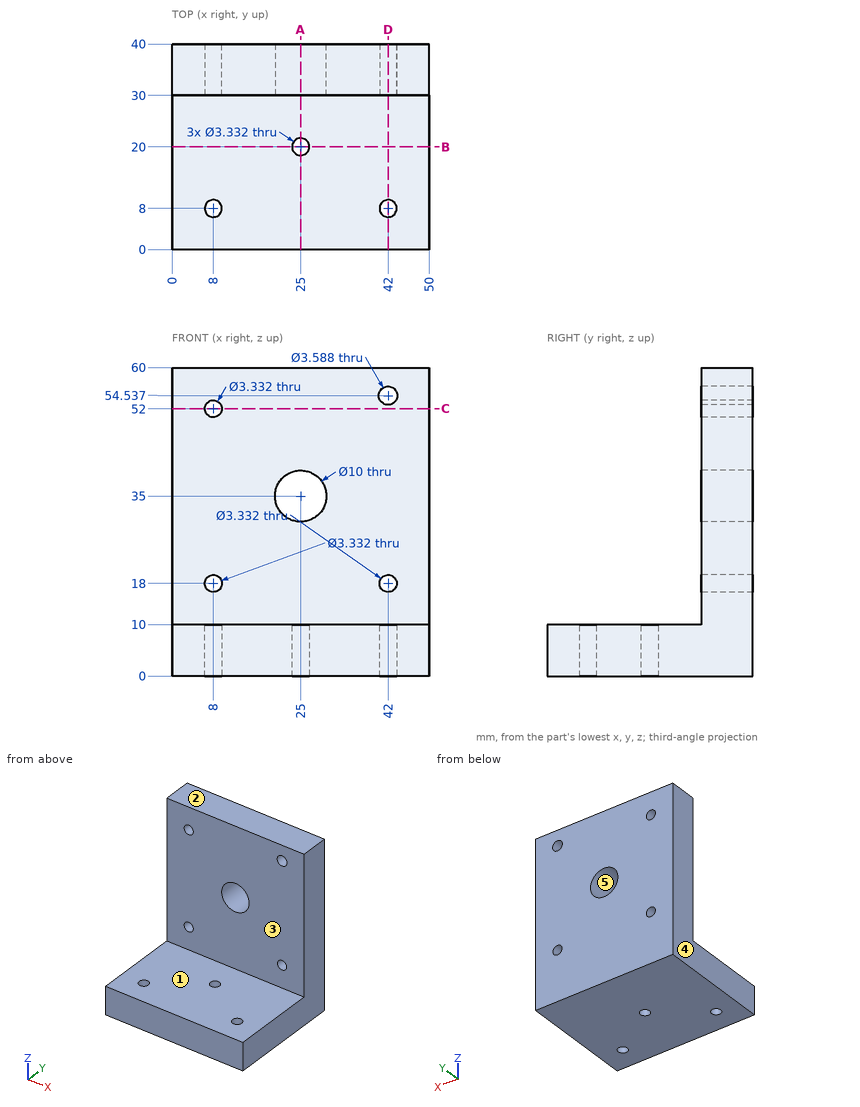
Design review of the part shown in the three views and the two pictorial views. Dimensions are in mm from the part's minimum x, y and z. A direction names the side the tool comes from. Round coordinates to 2 decimals unless told otherwise and drop trailing zeros. Write each loop counter-clockwise with the first axis right and the second up, starting at its lowest first coordinate (ties: lowest second). Pieces come first, ordered by that corner, then holes. Notation, with made-up numbers: M -20.5,27.25 L -5.5,27.25 A21 ccw -5.5,45.25 Z; hole C -21.75,-23 d7. An arc over 180 degrees is marked long. One line per item, written item: value. Start each with the question number.
1. To check wall thickness, follow probe 1 along X at (y, z) = (37, 52); probe 2 along X at (y, z) = (9, 4); probe 3 along Z at (x, y) = (25, 35). State the ranges of each line that lie inside material, in increasing order. Write a range as from..to.
2. Take a section at A-A on x = 25. State the section outline as (y, z) points.
3. Clearance check with flat-ended pins moving along their axes: P1, Ø4.5, axis at x = 42, z = 18, coming from the -Y side; P2, Ø4, axis at x = 35.5, y = 8, coming from the +Z side. State where each tip first meets the part, or that it passes through.
4. Take a section at D-D on x = 42. State the section outline as (y, z) points.
5. Take a section at C-C on z = 52. State the section outline as (x, y) points, then the cut area to 3 significant figures.
6. Draft analysis for pull direction X (two halves, no side actions). For the marked faces 3, 4 and 5, state which applies: pulls with the +X half, pulls with the -X half, needs draft (parallel to the pull), parting line crosses it, or undercut.
7. Take a section at B-B on y = 20. State the section outline as (x, z) points.
8. For the marked faces 1 and 2, list the 3-axis set-ups (+Z, -Z, +X, -X, +Y, -Y) from which the entire face can be reached by the end or side of a thin tool; tool diameter is ignored.
Computed:
1. probe 1: x = 0..6.33, 9.67..50
1. probe 2: x = 0..6.67, 9.33..40.67, 43.33..50
1. probe 3: z = 0..30, 40..60
2. outline: M 0,0 L 18.33,0 L 18.33,10 L 0,10 Z; M 21.67,0 L 40,0 L 40,30 L 30,30 L 30,10 L 21.67,10 Z; M 30,40 L 40,40 L 40,60 L 30,60 Z
3. P1: stops at y = 30
3. P2: stops at z = 10
4. outline: M 0,0 L 6.33,0 L 6.33,10 L 0,10 Z; M 9.67,0 L 40,0 L 40,16.33 L 30,16.33 L 30,10 L 9.67,10 Z; M 30,19.67 L 40,19.67 L 40,52.74 L 30,52.74 Z; M 30,56.33 L 40,56.33 L 40,60 L 30,60 Z
5. outline: M 0,30 L 6.33,30 L 6.33,40 L 0,40 Z; M 9.67,30 L 50,30 L 50,40 L 9.67,40 Z
5. area: 467 mm²
6. face 3: needs draft
6. face 4: pulls with the -X half
6. face 5: undercut
7. outline: M 0,0 L 23.33,0 L 23.33,10 L 0,10 Z; M 26.67,0 L 50,0 L 50,10 L 26.67,10 Z
8. face 1: +Z, +X, -X, -Y
8. face 2: +Z, +X, -X, +Y, -Y
